Verification items for the finished model (mm, model axes). Face numbers are marked on the shaded views. A direction names the side the tool comes from. Round coordinates to 2 decimals unless told otherwise and drop trailing zeros. Write each loop counter-clockwise with the first axis right and the second up, starting at its lowest first coordinate (ties: lowest second). Pieces come first, ordered by that corner, then holes.
from build123d import *

# Parameters (mm, degrees)
BOSS_EXTRUDE1_DEPTH            = 52.45
F_4_40_TAPPED_HOLE1_D          = 2.2606
SKETCH14_W                     = 80
SKETCH14_H                     = 8.065
BOSS_EXTRUDE2_DEPTH            = 8
SKETCH19_W                     = 80
SKETCH19_H                     = 68.58
BOSS_EXTRUDE3_DEPTH            = 8.5
CBORE_FOR_M6_SHCS2_D           = 6.6
CBORE_FOR_M6_SHCS2_CBORE_D     = 11
CBORE_FOR_M6_SHCS2_CBORE_DEPTH = 6
CHAMFER1_SIZE                  = 10
CHAMFER2_SIZE                  = 10
CHAMFER3_SIZE                  = 10


with BuildPart() as part:
    # Sketch1 → Boss-Extrude1 (new body)
    with BuildSketch(Plane(origin=(0, 0, 0), x_dir=(1, 0, 0), z_dir=(0, 1, 0))):
        Polygon((74.5, 8), (74.5, -90), (44.5, -120), (-44.5, -120), (-74.5, -90), (-74.5, 8), (-223, 8), (-223, 0), (-82.5, 0), (-82.5, -93.313708499), (-47.813708499, -128), (47.813708499, -128), (82.5, -93.313708499), (82.5, 0), (223, 0), (223, 8), align=None)
    extrude(amount=BOSS_EXTRUDE1_DEPTH)

    # #4-40 Tapped Hole1 (through all)
    with Locations(Plane(origin=(0, 0, 120), x_dir=(-1, 0, 0), z_dir=(0, 0, -1))):
        with Locations((-37.5, 38.725), (-37.5, 13.725), (37.5, 13.725), (37.5, 38.725), (-25.4, 26.225), (25.4, 26.225)):
            Hole(F_4_40_TAPPED_HOLE1_D / 2)

    # Sketch14 → Boss-Extrude2 (add)
    with BuildSketch(Plane(origin=(0, 0, -8), x_dir=(-1, 0, 0), z_dir=(0, 0, -1))):
        with Locations((-183, 56.4825)):
            Rectangle(SKETCH14_W, SKETCH14_H)
        with Locations((-183, -4.0325)):
            Rectangle(SKETCH14_W, SKETCH14_H)
        with Locations((183, -4.0325)):
            Rectangle(SKETCH14_W, SKETCH14_H)
        with Locations((183, 56.4825)):
            Rectangle(SKETCH14_W, SKETCH14_H)
    extrude(amount=-BOSS_EXTRUDE2_DEPTH)

    # Sketch19 → Boss-Extrude3 (add)
    with BuildSketch(Plane.XY):
        with Locations((-183, 26.225)):
            Rectangle(SKETCH19_W, SKETCH19_H)
        with Locations((183, 26.225)):
            Rectangle(SKETCH19_W, SKETCH19_H)
    extrude(amount=BOSS_EXTRUDE3_DEPTH)

    # CBORE for M6 SHCS2 (through all)
    with Locations(Plane(origin=(0, 0, -8), x_dir=(-1, 0, 0), z_dir=(0, 0, -1))):
        with Locations((-201, 1.225), (-201, 26.225), (-201, 51.225), (201, 1.225), (201, 26.225), (201, 51.225), (-188.5, 51.225), (-213.5, 51.225), (-213.5, 1.225), (-213.5, 26.225), (-188.5, 26.225), (-188.5, 1.225), (188.5, 1.225), (188.5, 26.225), (188.5, 51.225), (213.5, 51.225), (213.5, 1.225), (213.5, 26.225)):
            CounterBoreHole(CBORE_FOR_M6_SHCS2_D / 2, CBORE_FOR_M6_SHCS2_CBORE_D / 2, CBORE_FOR_M6_SHCS2_CBORE_DEPTH)

    # Chamfer1
    # the kernel refuses this chamfer: 10 mm, written as the material it adds along each edge
    with BuildSketch(Plane(origin=(143, 52.45, -8), x_dir=(-0.9996219169112968, -0.027495876610586282, 0), z_dir=(0, 0, 1))) as chamfer1_piece_1_section:
        Polygon((CHAMFER1_SIZE * 0.999621916911, -CHAMFER1_SIZE * 0.0274958766106), (-CHAMFER1_SIZE * 0.0274958766106, -CHAMFER1_SIZE * 0.999621916911), (0, 0), align=None)
    chamfer1_piece_1 = extrude(amount=8, mode=Mode.PRIVATE)
    chamfer1_piece_1 = split(chamfer1_piece_1, bisect_by=Plane(origin=(139.550321437, 60.515, -4), z_dir=(0, -1, 0)), keep=Keep.TOP, mode=Mode.PRIVATE)
    add(chamfer1_piece_1)
    with BuildSketch(Plane(origin=(143, 0, -8), x_dir=(-0.9996219169112969, 0.027495876610581386, 0), z_dir=(0, 0, 1))) as chamfer1_piece_2_section:
        Polygon((CHAMFER1_SIZE * 0.999621916911, CHAMFER1_SIZE * 0.0274958766106), (-CHAMFER1_SIZE * 0.0274958766106, CHAMFER1_SIZE * 0.999621916911), (0, 0), align=None)
    chamfer1_piece_2 = extrude(amount=8, mode=Mode.PRIVATE)
    chamfer1_piece_2 = split(chamfer1_piece_2, bisect_by=Plane(origin=(139.550321437, -8.065, -4), z_dir=(0, 1, 0)), keep=Keep.TOP, mode=Mode.PRIVATE)
    add(chamfer1_piece_2)
    with BuildSketch(Plane(origin=(-143, 0, -8), x_dir=(0.9996219169112969, 0.027495876610581386, 0), z_dir=(0, 0, 1))) as chamfer1_piece_3_section:
        Polygon((CHAMFER1_SIZE * 0.999621916911, -CHAMFER1_SIZE * 0.0274958766106), (-CHAMFER1_SIZE * 0.0274958766106, -CHAMFER1_SIZE * 0.999621916911), (0, 0), align=None)
    chamfer1_piece_3 = extrude(amount=8, mode=Mode.PRIVATE)
    chamfer1_piece_3 = split(chamfer1_piece_3, bisect_by=Plane(origin=(-139.550321437, -8.065, -4), z_dir=(0, 1, 0)), keep=Keep.TOP, mode=Mode.PRIVATE)
    add(chamfer1_piece_3)
    with BuildSketch(Plane(origin=(-143, 52.45, -8), x_dir=(0.9996219169112968, -0.027495876610586282, 0), z_dir=(0, 0, 1))) as chamfer1_piece_4_section:
        Polygon((CHAMFER1_SIZE * 0.999621916911, CHAMFER1_SIZE * 0.0274958766106), (-CHAMFER1_SIZE * 0.0274958766106, CHAMFER1_SIZE * 0.999621916911), (0, 0), align=None)
    chamfer1_piece_4 = extrude(amount=8, mode=Mode.PRIVATE)
    chamfer1_piece_4 = split(chamfer1_piece_4, bisect_by=Plane(origin=(-139.550321437, 60.515, -4), z_dir=(0, -1, 0)), keep=Keep.TOP, mode=Mode.PRIVATE)
    add(chamfer1_piece_4)

    # Chamfer2
    # the kernel refuses this chamfer: 10 mm, written as the material it adds along each edge
    with BuildSketch(Plane(origin=(143, -8.065, 0), x_dir=(0.027495876610908077, 0, 0.9996219169112879), z_dir=(0, 1, 0))) as chamfer2_piece_1_section:
        Polygon((CHAMFER2_SIZE * 0.999621916911, -CHAMFER2_SIZE * 0.0274958766106), (-CHAMFER2_SIZE * 0.0274958766109, -CHAMFER2_SIZE * 0.999621916911), (0, 0), align=None)
    chamfer2_piece_1 = extrude(amount=68.58, mode=Mode.PRIVATE)
    chamfer2_piece_1 = split(chamfer2_piece_1, bisect_by=Plane(origin=(140.422114736, -3.467675987, 8.5), z_dir=(0, 0, -1)), keep=Keep.TOP, mode=Mode.PRIVATE)
    chamfer2_piece_1 = split(chamfer2_piece_1, bisect_by=Plane(origin=(138.444895362, -5.444895362, 3.487912503), z_dir=(0.7071067811868302, 0.7071067811862648, 0)), keep=Keep.TOP, mode=Mode.PRIVATE)
    chamfer2_piece_1 = split(chamfer2_piece_1, bisect_by=Plane(origin=(140.422114736, 0, 3.487912503), z_dir=(0, -1, 0)), keep=Keep.TOP, mode=Mode.PRIVATE)
    add(chamfer2_piece_1)
    with BuildSketch(Plane(origin=(143, -8.065, 0), x_dir=(0.027495876610908077, 0, 0.9996219169112879), z_dir=(0, 1, 0))) as chamfer2_piece_2_section:
        Polygon((CHAMFER2_SIZE * 0.999621916911, -CHAMFER2_SIZE * 0.0274958766106), (-CHAMFER2_SIZE * 0.0274958766109, -CHAMFER2_SIZE * 0.999621916911), (0, 0), align=None)
    chamfer2_piece_2 = extrude(amount=68.58, mode=Mode.PRIVATE)
    chamfer2_piece_2 = split(chamfer2_piece_2, bisect_by=Plane(origin=(139.596737512, 52.45, 3.097187729), z_dir=(0, -1, 0)), keep=Keep.TOP, mode=Mode.PRIVATE)
    chamfer2_piece_2 = split(chamfer2_piece_2, bisect_by=Plane(origin=(139.596737512, 26.225, 8.5), z_dir=(0, 0, -1)), keep=Keep.TOP, mode=Mode.PRIVATE)
    chamfer2_piece_2 = split(chamfer2_piece_2, bisect_by=Plane(origin=(139.596737512, 0, 3.097187729), z_dir=(0, 1, 0)), keep=Keep.TOP, mode=Mode.PRIVATE)
    add(chamfer2_piece_2)
    with BuildSketch(Plane(origin=(143, -8.065, 0), x_dir=(0.027495876610908077, 0, 0.9996219169112879), z_dir=(0, 1, 0))) as chamfer2_piece_3_section:
        Polygon((CHAMFER2_SIZE * 0.999621916911, -CHAMFER2_SIZE * 0.0274958766106), (-CHAMFER2_SIZE * 0.0274958766109, -CHAMFER2_SIZE * 0.999621916911), (0, 0), align=None)
    chamfer2_piece_3 = extrude(amount=68.58, mode=Mode.PRIVATE)
    chamfer2_piece_3 = split(chamfer2_piece_3, bisect_by=Plane(origin=(140.422114736, 52.45, 3.487912503), z_dir=(0, 1, 0)), keep=Keep.TOP, mode=Mode.PRIVATE)
    chamfer2_piece_3 = split(chamfer2_piece_3, bisect_by=Plane(origin=(140.422114736, 55.917675987, 8.5), z_dir=(0, 0, -1)), keep=Keep.TOP, mode=Mode.PRIVATE)
    chamfer2_piece_3 = split(chamfer2_piece_3, bisect_by=Plane(origin=(138.444895362, 57.894895362, 3.487912503), z_dir=(0.7071067811868302, -0.7071067811862648, 0)), keep=Keep.TOP, mode=Mode.PRIVATE)
    add(chamfer2_piece_3)

    # Chamfer3
    # the kernel refuses this chamfer: 10 mm, written as the material it adds along each edge
    with BuildSketch(Plane(origin=(-143, 60.515, 0), x_dir=(-0.027495876610908083, 0, 0.9996219169112879), z_dir=(0, -1, 0))) as chamfer3_piece_1_section:
        Polygon((CHAMFER3_SIZE * 0.999621916911, -CHAMFER3_SIZE * 0.0274958766106), (-CHAMFER3_SIZE * 0.0274958766109, -CHAMFER3_SIZE * 0.999621916911), (0, 0), align=None)
    chamfer3_piece_1 = extrude(amount=68.58, mode=Mode.PRIVATE)
    chamfer3_piece_1 = split(chamfer3_piece_1, bisect_by=Plane(origin=(-140.422114736, 55.917675987, 8.5), z_dir=(0, 0, -1)), keep=Keep.TOP, mode=Mode.PRIVATE)
    chamfer3_piece_1 = split(chamfer3_piece_1, bisect_by=Plane(origin=(-138.444895362, 57.894895362, 3.487912503), z_dir=(-0.7071067811868302, -0.7071067811862648, 0)), keep=Keep.TOP, mode=Mode.PRIVATE)
    chamfer3_piece_1 = split(chamfer3_piece_1, bisect_by=Plane(origin=(-140.422114736, 52.45, 3.487912503), z_dir=(0, 1, 0)), keep=Keep.TOP, mode=Mode.PRIVATE)
    add(chamfer3_piece_1)
    with BuildSketch(Plane(origin=(-143, 60.515, 0), x_dir=(-0.027495876610908083, 0, 0.9996219169112879), z_dir=(0, -1, 0))) as chamfer3_piece_2_section:
        Polygon((CHAMFER3_SIZE * 0.999621916911, -CHAMFER3_SIZE * 0.0274958766106), (-CHAMFER3_SIZE * 0.0274958766109, -CHAMFER3_SIZE * 0.999621916911), (0, 0), align=None)
    chamfer3_piece_2 = extrude(amount=68.58, mode=Mode.PRIVATE)
    chamfer3_piece_2 = split(chamfer3_piece_2, bisect_by=Plane(origin=(-139.596737512, 0, 3.097187729), z_dir=(0, 1, 0)), keep=Keep.TOP, mode=Mode.PRIVATE)
    chamfer3_piece_2 = split(chamfer3_piece_2, bisect_by=Plane(origin=(-139.596737512, 26.225, 8.5), z_dir=(0, 0, -1)), keep=Keep.TOP, mode=Mode.PRIVATE)
    chamfer3_piece_2 = split(chamfer3_piece_2, bisect_by=Plane(origin=(-139.596737512, 52.45, 3.097187729), z_dir=(0, -1, 0)), keep=Keep.TOP, mode=Mode.PRIVATE)
    add(chamfer3_piece_2)
    with BuildSketch(Plane(origin=(-143, 60.515, 0), x_dir=(-0.027495876610908083, 0, 0.9996219169112879), z_dir=(0, -1, 0))) as chamfer3_piece_3_section:
        Polygon((CHAMFER3_SIZE * 0.999621916911, -CHAMFER3_SIZE * 0.0274958766106), (-CHAMFER3_SIZE * 0.0274958766109, -CHAMFER3_SIZE * 0.999621916911), (0, 0), align=None)
    chamfer3_piece_3 = extrude(amount=68.58, mode=Mode.PRIVATE)
    chamfer3_piece_3 = split(chamfer3_piece_3, bisect_by=Plane(origin=(-140.422114736, 0, 3.487912503), z_dir=(0, -1, 0)), keep=Keep.TOP, mode=Mode.PRIVATE)
    chamfer3_piece_3 = split(chamfer3_piece_3, bisect_by=Plane(origin=(-140.422114736, -3.467675987, 8.5), z_dir=(0, 0, -1)), keep=Keep.TOP, mode=Mode.PRIVATE)
    chamfer3_piece_3 = split(chamfer3_piece_3, bisect_by=Plane(origin=(-138.444895362, -5.444895362, 3.487912503), z_dir=(-0.7071067811868302, 0.7071067811862648, 0)), keep=Keep.TOP, mode=Mode.PRIVATE)
    add(chamfer3_piece_3)


solid = part.part
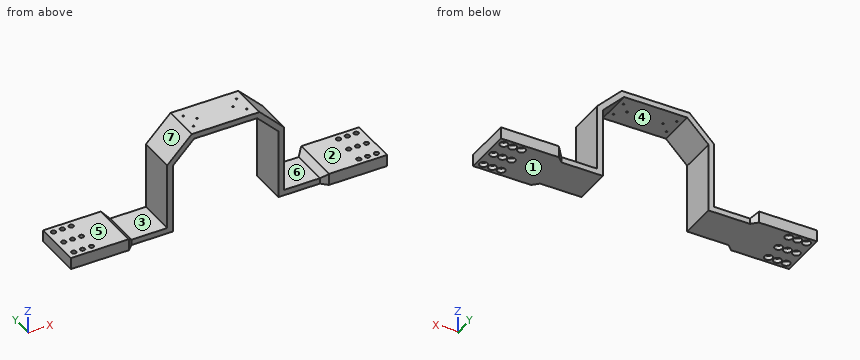
Q1. Sectioned sample at A-A (z = 53.5). Enter the section's corners in (x, y).
Recorded:
outline: (-82.5, 0) - (-74.5, 0) - (-74.5, 52.45) - (-82.5, 52.45) - close; (74.5, 0) - (82.5, 0) - (82.5, 52.45) - (74.5, 52.45) - close
Q2. Release check for a two-part mould opening along X. For the marked faces 5, 6 and 7 record: released by +X, released by -X, zero draft, split by the parting line, or undercut.
Recorded:
face 5: zero draft
face 6: undercut
face 7: released by -X
Q3. Tool access check on the marked faces 1, 2, 3 and 4. Record the directions out of +Z, -Z, +X, -X, +Y, -Y that give a thin tool (end or side, any length) a straight path to the whole face; none if there is none.
Recorded:
face 1: -Z, +X, -X, +Y, -Y
face 2: +Z, +X, +Y, -Y
face 3: +Z, +Y, -Y
face 4: -Z, +Y, -Y
Q4. Depth check by flat-ended pin: P1, Ø12.5, axis at x = 188.5, y = 1.225, coming from the +Z side; P2, Ø3, axis at x = -25.4, y = 26.225, coming from the -Z side; P3, Ø6, axis at x = -201, y = 1.225, coming from the -Z side; P4, Ø6, axis at x = -69, y = 2.5, coming from the +Z side. Enter the tip coordinate at first touch or a pass-through.
Recorded:
P1: stops at z = 8.5
P2: stops at z = 120
P3: passes through
P4: stops at z = 109.81
Q5. Sectioned sample at B-B (x = 16). Enter the section's corners in (y, z).
Recorded:
outline: (0, 120) - (52.45, 120) - (52.45, 128) - (0, 128) - close
Q6. Material ranges on line 1 along Y through (x, z) = (188, 2) (3 decimals); line 2 along Y through (x, z) = (201, -6) (3 decimals); line 3 along Y through (x, z) = (37, 122), recorded low to high.
Recorded:
line 1: y = -8.065 to -2.037, 4.487 to 22.963, 29.487 to 47.963, 54.487 to 60.515
line 2: y = -8.065 to -4.275, 6.725 to 20.725, 31.725 to 45.725, 56.725 to 60.515
line 3: y = 0 to 12.71, 14.74 to 37.71, 39.74 to 52.45
